Autodesk Inventor part; units mm, degrees
ref_plane "YZ Plane" through (0, 0, 0) normal (1, 0, 0) x (0, 1, 0)
ref_plane "XZ Plane" through (0, 0, 0) normal (0, 1, 0) x (-1, 0, 0)
ref_plane "XY Plane" through (0, 0, 0) normal (0, 0, 1) x (1, 0, 0)
sketch "Sketch1" plane through (0, 0, 0) normal (0, 0, 1) x (1, 0, 0)
  line L0 (0, 0) -> (-17.8576, 0)
  line L1 (-17.8576, 0) -> (-17.8576, 11.024)
  line L2 (-17.8576, 11.024) -> (0, 11.024)
  line L3 (0, 11.024) -> (0, 0)
extrude "Extrusion1" add sketch "Sketch1" along normal blind 12.7
sketch "Sketch2" plane through (-17.8576, 11.024, 0) normal (0, 1, 0) x (1, 0, 0)
  circle A0 centre (13.7961, -8.2519) radius 1.3228
  circle A1 centre (5.0929, -8.2519) radius 1.3477
  line L0 (12.4733, -4.1259) -> (6.4406, -4.1259)
  line L1 (6.4406, -4.1259) -> (6.4406, -1.4183)
  line L2 (6.4406, -1.4183) -> (12.4733, -1.4183)
  line L3 (12.4733, -1.4183) -> (12.4733, -4.1259)
  point P0 (17.8576, 0)
extrude "Extrusion2" cut sketch "Sketch2" against normal blind 2.54
fillet "Fillet1" radius 3.175 1 edges at (-17.8576, 5.512, 12.7)
fillet "Fillet2" radius 3.175 1 edges at (-17.8576, 5.512, 0)
fillet "Fillet3" radius 3.175 1 edges at (0, 5.512, 12.7)
fillet "Fillet4" radius 3.175 1 edges at (0, 5.512, 0)
sketch "Sketch3" plane through (0, 0, 0) normal (0, 0, -1) x (-1, 0, 0)
  circle A0 centre (8.0161, 5.0375) radius 2.5669
  point P0 (0, 0)
extrude "Extrusion3" cut sketch "Sketch3" against normal blind 7.62
sketch "Sketch4" plane through (0, 0, 12.7) normal (0, 0, 1) x (1, 0, 0)
  circle A0 centre (-9.0674, 5.2127) radius 2.2357
  point P0 (0, 0)
extrude "Extrusion4" add sketch "Sketch4" along normal blind 2.54
properties part number "finalface4"
Geometry: final body of the model. Coordinates: model frame, mm. A direction names the side the tool comes from. Coordinates: 2 decimals unless noted, no trailing zeros. Order: outer loops, then holes, each group sorted by start corner. A loop starts at its lowest first (then second) coordinate and runs counter-clockwise, first axis right, second up. Notation, with made-up numbers: (4.25, -12) -> (50.25, -12) arc R8 cw to (50.25, 1) -> close; hole circle Ø5 at (65.5, 45). An arc over 180 degrees is marked (long way). Write each question's results on one line, items separated by ' | '. Start each with the question number.
1) Material intervals for line 1 along X through (y, z) = (5, 4.5); line 2 along Z through (x, y) = (-9.5, 10.5); line 3 along Y through (x, z) = (-9, 13), sorted ascending.
2) First-contact query: pin 1 (4 mm diameter, centred on x = -4.06, z = 8.25, fed in from +Y); pin 2 (3 mm diameter, centred on x = -7.5, y = 10.5, fed in from +Z); pin 3 (4.5 mm diameter, centred on x = -8.02, y = 5.04, fed in from -Z); pin 4 (0.8 mm diameter, centred on x = -9, z = 2.5, fed in from +Y). Flat tips, straight axial feed; report the tip coordinate or a pass-through.
3) Cut plane C-C, the plane x = -13. Output: boundary loops of the cut face in (y, z).
4) Cut plane B-B, the plane z = 2. Output: boundary loops of the cut face in (x, y).
5) Cut plane A-A, the plane y = 1. Output: boundary loops of the cut face in (x, z) (3 decimals).
6) Set-up query: faces 5 (the flat face through (-8, 10, 4.126)), 6 (the flat face through (-8, 5, 7.62)), 7 (the flat face through (-9, 0, 6)). Return all of +Z, -Z, +X, -X, +Y, -Y with unobstructed straight access to the full face (end or side cutting, diameter ignored); none if empty.
7) Cut plane D-D, the plane y = 10. State how many separate pieces and enclosed holes the cut face has, and give its area (3 significant figures).
8) Mould query, pull axis Z, two halves, no side actions, for faces 1 (the flat face through (-11.417, 10, 3)), 2 (the cylindrical face through (-7.002, 6.069, 13.952)), 3 (the flat face through (-13, 8.484, 8)), 4 (the flat face through (-9, 8, 12.7)). Classes: released by +Z, released by -Z, zero draft, split by the parting line, or undercut.
Checks:
1) line 1: -17.86 to -10.58, -5.45 to 0 | line 2: 0 to 1.42, 4.13 to 12.7 | line 3: 2.98 to 7.45
2) pin 1: y = 11.02 | pin 2: z = 12.7 | pin 3: z = 7.62 | pin 4: y = 8.48
3) outline: (0, 0) -> (11.02, 0) -> (11.02, 6.92) -> (8.48, 6.92) -> (8.48, 9.58) -> (11.02, 9.58) -> (11.02, 12.7) -> (0, 12.7) -> close
4) outline: (-17.63, 0) -> (-0.23, 0) -> (-0.23, 11.02) -> (-5.38, 11.02) -> (-5.38, 8.48) -> (-11.42, 8.48) -> (-11.42, 11.02) -> (-17.63, 11.02) -> close; hole circle Ø5.13 at (-8.02, 5.04)
5) outline: (-17.858, 3.175) arc R3.175 ccw to (-14.683, 0) -> (-3.175, 0) arc R3.175 ccw to (0, 3.175) -> (0, 9.525) arc R3.175 ccw to (-3.175, 12.7) -> (-14.683, 12.7) arc R3.175 ccw to (-17.858, 9.525) -> close
6) face 5: +Y | face 6: -Z | face 7: +Z, -Z, +X, -X, -Y
7) separate pieces: 1 | enclosed holes: 3 | area: 191 mm^2
8) face 1: undercut | face 2: zero draft | face 3: undercut | face 4: released by +Z
